```python
from build123d import *

# Parameters (mm, degrees)
SKETCH_1_W          = 36
SKETCH_1_H          = 18
EXTRUDE_1_DEPTH     = 3
SKETCH_2_W          = 8
SKETCH_2_H          = 5
EXTRUDE_2_DEPTH     = 10
EXTRUDE_3_DEPTH     = 11
SKETCH_4_W          = 25
SKETCH_4_H          = 4
CUT_EXTRUDE_1_DEPTH = 4


with BuildPart() as part:
    # 草图1 → 凸台-拉伸1 (new body)
    with BuildSketch(Plane(origin=(0, 0, 0), x_dir=(1, 0, 0), z_dir=(0, 1, 0))):
        Rectangle(SKETCH_1_W, SKETCH_1_H)
    extrude(amount=EXTRUDE_1_DEPTH)

    # 草图2 → 凸台-拉伸2 (add)
    with BuildSketch(Plane(origin=(0, 3, 0), x_dir=(1, 0, 0), z_dir=(0, 1, 0))):
        with Locations((-14, -6.5)):
            Rectangle(SKETCH_2_W, SKETCH_2_H)
        with Locations((14, -6.5)):
            Rectangle(SKETCH_2_W, SKETCH_2_H)
    extrude(amount=EXTRUDE_2_DEPTH)

    # 草图3 → 凸台-拉伸3 (add)
    with BuildSketch(Plane(origin=(0, 3, 0), x_dir=(1, 0, 0), z_dir=(0, 1, 0))):
        Polygon((-18, 9), (-18, -4), (-12.5, -4), (-12.5, 5), (12.5, 5), (12.5, -4), (18, -4), (18, 9), align=None)
    extrude(amount=EXTRUDE_3_DEPTH)

    # 草图4 → 切除-拉伸1 (cut)
    with BuildSketch(Plane(origin=(0, 14, 0), x_dir=(1, 0, 0), z_dir=(0, 1, 0))):
        with Locations((0, 7)):
            Rectangle(SKETCH_4_W, SKETCH_4_H)
    extrude(amount=-CUT_EXTRUDE_1_DEPTH, mode=Mode.SUBTRACT)


solid = part.part
```
The model under review builds one solid part; all positions refer to its coordinate system, in mm. A direction names the side the tool comes from. Round coordinates to 2 decimals unless told otherwise and drop trailing zeros. Loops run counter-clockwise (first coordinate to the right, second up) from the corner with the lowest first, then second, coordinate; pieces in that order, holes last.
1) Consider section B-B on z = -4.5. State the section outline as (x, y) points, then the cut area to 3 significant figures.
Values follow:
outline: (-18, 0) - (18, 0) - (18, 14) - (12.5, 14) - (12.5, 3) - (-12.5, 3) - (-12.5, 14) - (-18, 14) - close
area: 229 mm2
2) Consider section A-A on y = 11.75. State the section outline as (x, z) points.
Values follow:
outline: (-18, -9) - (-12.5, -9) - (-12.5, 4) - (-10, 4) - (-10, 9) - (-18, 9) - close; (10, 4) - (12.5, 4) - (12.5, -9) - (18, -9) - (18, 9) - (10, 9) - close
3) Consider section D-D on x = 10.5. State the section outline as (y, z) points.
Values follow:
outline: (0, -9) - (10, -9) - (10, -5) - (3, -5) - (3, 4) - (13, 4) - (13, 9) - (0, 9) - close
4) Tool access review of faces 5 (the face through (12.5, 9, -1)), 6 (the face through (0, 10, -7)), 7 (the face through (15.2, 13.5, 4)): name each direction out of +Z, -Z, +X, -X, +Y, -Y from which nothing blocks a thin tool from reaching the whole face with its end or side.
Values follow:
face 5: +Y
face 6: -Z, +Y
face 7: +Z, +X, -X, +Y
5) The part is to be moulded in two halves that separate along X. For faces 1 (the face through (-12.5, 9, -1)), 2 (the face through (-18, 7, 0)), 3 (the face through (-15.3, 13.5, 4)), 4 (the face through (-10, 8, 7)), say which applies: pulls with the +X half, pulls with the -X half, needs draft (parallel to the pull), parting line crosses it, or undercut.
Values follow:
face 1: undercut
face 2: pulls with the -X half
face 3: needs draft
face 4: undercut
6) Consider section C-C on y = 9. State the section outline as (x, z) points, then the cut area to 3 significant figures.
Values follow:
outline: (-18, -9) - (18, -9) - (18, 9) - (10, 9) - (10, 4) - (12.5, 4) - (12.5, -5) - (-12.5, -5) - (-12.5, 4) - (-10, 4) - (-10, 9) - (-18, 9) - close
area: 323 mm2
7) Clearance check with flat-ended pins moving along their axes: P1, Ø1.5, axis at x = 1, z = -4, coming from the -Y side; P2, Ø3, axis at x = -4, z = -7, coming from the +Y side; P3, Ø4, axis at x = -4, z = 0.5, coming from the +Y side; P4, Ø0.5, axis at x = 15, y = 13.5, coming from the +Z side. State where each tip first meets the part, or that it passes through.
Values follow:
P1: stops at y = 0
P2: stops at y = 10
P3: stops at y = 3
P4: stops at z = 4
8) Wall thickness on line 1 along X through (y, z) = (13, -7.5); line 2 along Z through (x, y) = (6, 9.25); line 3 along Y through (x, z) = (7, -0.5): over which ranges is each line inside the solid? List them lowest first.
Values follow:
line 1: x = -18 to -12.5, 12.5 to 18
line 2: z = -9 to -5
line 3: y = 0 to 3
